```python
from build123d import *

# Parameters (mm, degrees)
F0_W     = 203
F0_H     = 140
F1_DEPTH = 45
F2_W     = 195
F2_H     = 56
F3_DEPTH = 41
F4_R     = 16.5
F5_DEPTH = 41
F6_R     = 10
F7_R     = 5


with BuildPart() as f1:
    # F0 (on Top) → F1 (new body)
    with BuildSketch(Plane.XY):
        Rectangle(F0_W, F0_H)
    extrude(amount=F1_DEPTH)

    # F2 (on face) → F3 (cut)
    with BuildSketch(Plane.XY.offset(45)):
        with Locations((0, 38)):
            Rectangle(F2_W, F2_H)
    extrude(amount=-F3_DEPTH, mode=Mode.SUBTRACT)

    # F4 (on face) → F5 (cut)
    with BuildSketch(Plane.XY.offset(45)):
        with BuildLine():
            ThreePointArc((-42.7083130081, 10), (-13.5015619392, -64.1425780905), (50, -16))
            ThreePointArc((50, -16), (48.1425780905, -2.4984380608), (42.7083130081, 10))
            Line((42.7083130081, 10), (-42.7083130081, 10))
        make_face()
        with Locations((0, -16)):
            Circle(F4_R, mode=Mode.SUBTRACT)
    extrude(amount=-F5_DEPTH, mode=Mode.SUBTRACT)

    # F6
    f6_edges = [f1.edges().sort_by_distance(p)[0] for p in [
        (97.5, 66, 24.5),
        (-97.5, 66, 24.5),
        (97.5, 10, 24.5),
        (-97.5, 10, 24.5),
    ]]
    fillet(f6_edges, radius=F6_R)

    # F7
    f7_edges = [f1.edges().sort_by_distance(p)[0] for p in [
        (42.708313, 10, 24.5),
        (-42.708313, 10, 24.5),
    ]]
    fillet(f7_edges, radius=F7_R)


solid = f1.part
```
The model under review builds one solid part; all positions refer to its coordinate system, in mm. A direction names the side the tool comes from. Coordinates: 2 decimals unless noted, no trailing zeros. Order: outer loops, then holes, each group sorted by start corner. A loop starts at its lowest first (then second) coordinate and runs counter-clockwise, first axis right, second up. Notation, with made-up numbers: M 42,-6 L 96,-6 A20 cw 96,2 Z; hole C 39.25,18.5 d1. An arc over 180 degrees is marked long. One line per question, with ' | ' between items.
(1) Add section A-A, the plane z = 19.5. Write out the cut boundary in (x, y).
Geometry results:
outline: M -101.5,-70 L 101.5,-70 L 101.5,70 L -101.5,70 Z; C 0,-16 d33; hole M -97.5,20 A10 ccw -87.5,10 L -50.83,10 A5 cw -46.21,3.09 A50 ccw long 46.21,3.09 A5 cw 50.83,10 L 87.5,10 A10 ccw 97.5,20 L 97.5,56 A10 ccw 87.5,66 L -87.5,66 A10 ccw -97.5,56 Z
(2) The part is to be moulded in two halves that separate along Y. For faces 1 (the face through (-1, 70, 22)), 2 (the face through (-1, -70, 22)), 3 (the face through (-46.72, 7.84, 24.21)), 4 (the face through (69, 10, 25)), say which applies: +Y half, -Y half, draft (parallel to the pull), parting line (faces both ways), or undercut.
Geometry results:
face 1: +Y half | face 2: -Y half | face 3: undercut | face 4: undercut
(3) For probe 1 along Y at (x, z) = (0, 25); probe 2 along X at (y, z) = (-5.5, 17); probe 3 along X at (y, z) = (21, 21), list the stretches that pass through material, from the lowest coordinate up. Write a range as from..to.
Geometry results:
probe 1: y = -70..-66, -32.5..0.5, 66..70 | probe 2: x = -101.5..-48.89, -12.73..12.73, 48.89..101.5 | probe 3: x = -101.5..-97.5, 97.5..101.5
(4) Machinability: for faces 5 (the face through (-31, -57, 45)), 6 (the face through (-94.49, 12.85, 24.21)), which of the approach directions +Z, -Z, +X, -X, +Y, -Y give a long, thin tool a straight path to every point of the face, cutting with its end or side? Answer none if there is none.
Geometry results:
face 5: +Z, +X, -X, +Y, -Y | face 6: +Z
(5) Add section D-D, the plane x = 0. Write out the cut boundary in (y, z), then the cut area to 3 significant figures.
Geometry results:
outline: M -70,0 L 70,0 L 70,45 L 66,45 L 66,4 L 0.5,4 L 0.5,45 L -32.5,45 L -32.5,4 L -66,4 L -66,45 L -70,45 Z | area: 2,240 mm²
(6) Add section B-B, the plane x = -69.5. Write out the cut boundary in (y, z), then the cut area to 3 significant figures.
Geometry results:
outline: M -70,0 L 70,0 L 70,45 L 66,45 L 66,4 L 10,4 L 10,45 L -70,45 Z | area: 4,000 mm²
(7) Insertion check: pin 1 (8 mm diameter, centred on x = -36, y = -1.5, fed in from +Z). The pin has a flat end and moves straight along its axis. Give the tip position at first contact, or say it passes through.
Geometry results:
pin 1: stops at z = 4
(8) Add section C-C, the plane y = 30. Write out the cut boundary in (x, z), then the cut area to 3 significant figures.
Geometry results:
outline: M -101.5,0 L 101.5,0 L 101.5,45 L 97.5,45 L 97.5,4 L -97.5,4 L -97.5,45 L -101.5,45 Z | area: 1,140 mm²
